For this review, take the finished solid that the model builds, in its own axes (mm). Face numbers are marked on the shaded views. A direction names the side the tool comes from. Coordinates: 2 decimals unless noted, no trailing zeros. Write each loop counter-clockwise with the first axis right and the second up, starting at its lowest first coordinate (ties: lowest second). Pieces come first, ordered by that corner, then holes. Notation, with made-up numbers: M -32.5,84.5 L -28.5,84.5 A28 ccw -28.5,105.5 Z; hole C -16.75,83.25 d9. An arc over 180 degrees is marked long. Return JSON: item names as keys, results as strings.
```python
from build123d import *

# Parameters (mm, degrees)
SKETCH3_R           = 20.955
BOSS_EXTRUDE3_DEPTH = 3.81
SKETCH4_R           = 22.225
BOSS_EXTRUDE4_DEPTH = 34.29
SKETCH5_R           = 20.828
BOSS_EXTRUDE5_DEPTH = 27.432
SKETCH6_R           = 8.636
BOSS_EXTRUDE6_DEPTH = 4.064
SKETCH7_R           = 2.794
BOSS_EXTRUDE7_DEPTH = 16.002


with BuildPart() as part:
    # Sketch3 → Boss-Extrude3 (new body)
    with BuildSketch(Plane.XY):
        with Locations(Location((0, 0, 0), (0, 0, 180))):
            Circle(SKETCH3_R)
    extrude(amount=BOSS_EXTRUDE3_DEPTH)

    # Sketch4 → Boss-Extrude4 (add)
    with BuildSketch(Plane.XY.offset(3.81)):
        Circle(SKETCH4_R)
    extrude(amount=BOSS_EXTRUDE4_DEPTH)

    # Sketch5 → Boss-Extrude5 (add)
    with BuildSketch(Plane.XY.offset(38.1)):
        Circle(SKETCH5_R)
    extrude(amount=BOSS_EXTRUDE5_DEPTH)

    # Sketch6 → Boss-Extrude6 (add)
    with BuildSketch(Plane(origin=(0, 0, 0), x_dir=(-1, 0, 0), z_dir=(0, 0, -1))):
        Circle(SKETCH6_R)
    extrude(amount=BOSS_EXTRUDE6_DEPTH)

    # Sketch7 → Boss-Extrude7 (add)
    with BuildSketch(Plane(origin=(0, 0, -4.064), x_dir=(-1, 0, 0), z_dir=(0, 0, -1))):
        Circle(SKETCH7_R)
    extrude(amount=BOSS_EXTRUDE7_DEPTH)


solid = part.part
```
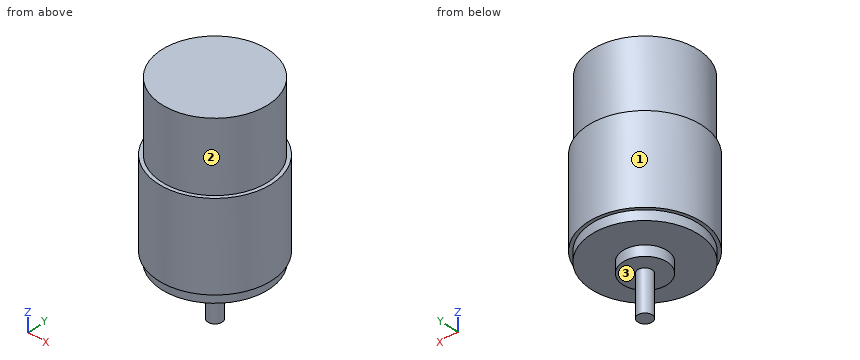
1. We need section D-D (x = 7). State the section outline as (y, z) points, plus the area to 3 significant figures.
Checks:
{"outline": "M -21.09,3.81 L -19.75,3.81 L -19.75,0 L -5.06,0 L -5.06,-4.06 L 5.06,-4.06 L 5.06,0 L 19.75,0 L 19.75,3.81 L 21.09,3.81 L 21.09,38.1 L 19.62,38.1 L 19.62,65.53 L -19.62,65.53 L -19.62,38.1 L -21.09,38.1 Z", "area": "2,710 mm2"}
2. We need section C-C (z = -1.5). State the section outline as (x, y) points, plus the area to 3 significant figures.
Checks:
{"outline": "C 0,0 d17.27", "area": "234 mm2"}
3. Wall thickness on L1, parallel to Z at x = -13.5, y = 17; L2, parallel to Z at x = 1.5, y = 13; L3, parallel to X at y = -2.5, z = 43: over which ranges is each line inside the solid? List them lowest first. Write a range as from..to.
Checks:
{"L1": "3.81..38.1", "L2": "0..65.53", "L3": "-20.68..20.68"}
4. We need section A-A (x = 0). State the section outline as (y, z) points (3 decimals).
Checks:
{"outline": "M -22.225,3.81 L -20.955,3.81 L -20.955,0 L -8.636,0 L -8.636,-4.064 L -2.794,-4.064 L -2.794,-20.066 L 2.794,-20.066 L 2.794,-4.064 L 8.636,-4.064 L 8.636,0 L 20.955,0 L 20.955,3.81 L 22.225,3.81 L 22.225,38.1 L 20.828,38.1 L 20.828,65.532 L -20.828,65.532 L -20.828,38.1 L -22.225,38.1 Z"}
5. Clearance check with flat-ended pins moving along their axes: pin 1 Ø4 at (x, y) = (-10.5, -5.5) entering from -Z; pin 2 Ø3 at (y, z) = (-5.5, 1) entering from +X; pin 3 Ø6 at (x, y) = (1, -6.5) entering from -Z. State where each tip first meets the part, or that it passes through.
Checks:
{"pin 1": "z = 0", "pin 2": "x = 20.57", "pin 3": "z = -4.06"}
6. For the marked faces 1, 2 and 3, list the 3-axis set-ups (+Z, -Z, +X, -X, +Y, -Y) from which the entire face can be reached by the end or side of a thin tool; tool diameter is ignored.
Checks:
{"face 1": "+Z, -Z", "face 2": "+Z", "face 3": "-Z"}
